Study the drawing (mm; zero at the part's minimum x, y, z) and answer. Coordinates: 2 decimals unless noted, no trailing zeros. Loops run counter-clockwise (first coordinate to the right, second up) from the corner with the lowest first, then second, coordinate; pieces in that order, holes last. Notation, with made-up numbers: (83, 55) - (119, 55) arc R20 ccw to (119, 72) - close; hole circle Ø9 at (55, -39.5). An arc over 180 degrees is marked (long way). Use one line per item in the form item = value.
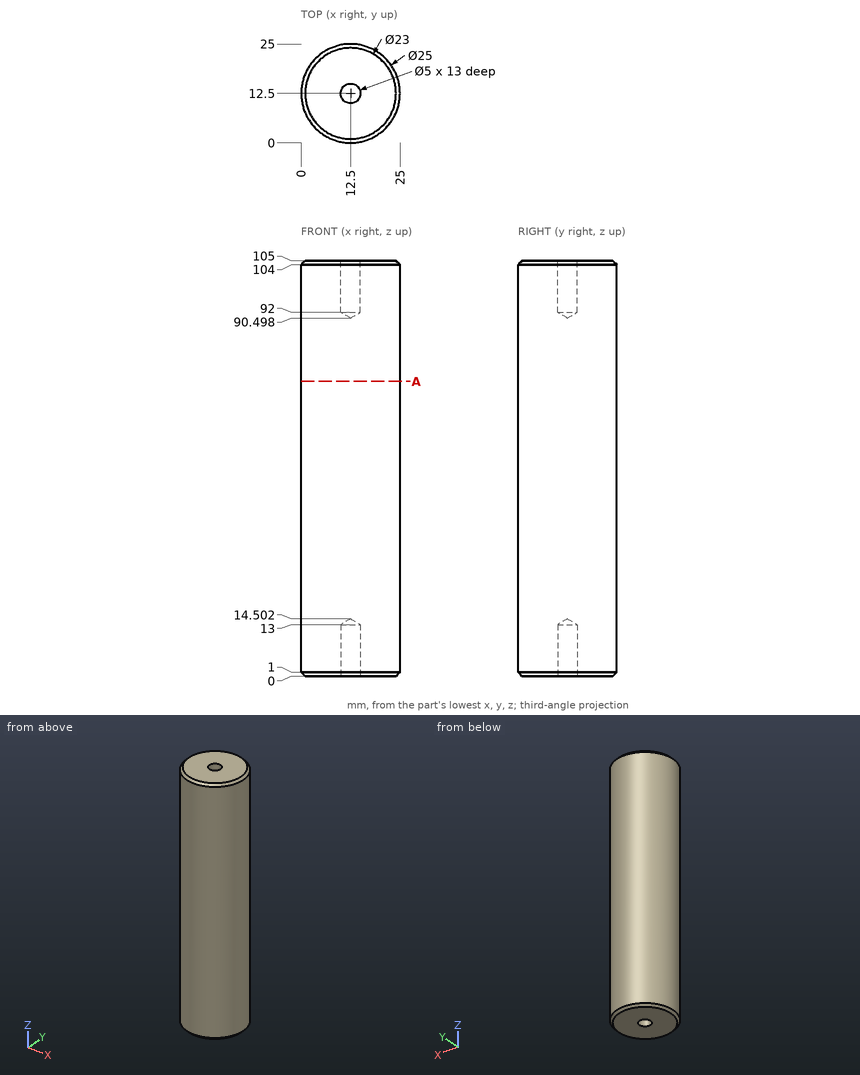
Item 1: Find the intervals of material crossed by L1, parallel to Y at x = 12.5, z = 7.75; L2, parallel to Y at x = 10.75, z = 96.5 (1 decimal); L3, parallel to X at y = 10.5, z = 94, in increasing order.
Results below:
L1 = 0 to 10, 15 to 25
L2 = 0.1 to 10.7, 14.3 to 24.9
L3 = 0.16 to 11, 14 to 24.84
Item 2: Each of these flat-tipped pins is pushed along its axis until it touches: P1, Ø6, axis at x = 20.5, z = 38, coming from the -Y side; P2, Ø6, axis at x = 12.5, y = 12.5, coming from the +Z side; P3, Ø1, axis at x = 10.5, z = 83.5, coming from the +Y side; P4, Ø3, axis at x = 3.5, z = 84.5, coming from the +Y side. Where does it stop, or does it pass through?
Results below:
P1 = 1.04
P2 = 105
P3 = 24.91
P4 = 22.5
Item 3: The part is cut by section A-A on z = 74.5. Give the vertices of the cut face in (x, y), plus the area to 3 significant figures.
Results below:
outline = circle Ø25 at (12.5, 12.5)
area = 491 mm²
